from build123d import *

# Parameters (mm, degrees)
SKETCH_1_R      = 1.05
SKETCH_1_R_2    = 1.585
SKETCH_1_W      = 25
SKETCH_1_H      = 2
EXTRUDE_1_DEPTH = 2


with BuildPart() as part:
    # 草图1 → 凸台-拉伸1 (new body)
    with BuildSketch(Plane(origin=(0, 0, 0), x_dir=(1, 0, 0), z_dir=(0, 1, 0))):
        Polygon((86.47, 0), (0, 0), (0, -8.9), (-8.17, -8.9), (-8.17, -15.78), (0, -15.78), (0, -34.06), (-8.17, -34.06), (-8.17, -42.03), (0, -42.03), (0, -115), (86.47, -115), align=None)
        with Locations(Location((3, -113, 0), (0, 0, 270))):
            Circle(SKETCH_1_R, mode=Mode.SUBTRACT)
        with Locations(Location((9.47, -87.2, 0), (0, 0, 270))):
            Circle(SKETCH_1_R_2, mode=Mode.SUBTRACT)
        with Locations(Location((53.97, -87.2, 0), (0, 0, 270))):
            Circle(SKETCH_1_R_2, mode=Mode.SUBTRACT)
        with Locations(Location((66, -113, 0), (0, 0, 270))):
            Circle(SKETCH_1_R, mode=Mode.SUBTRACT)
        with Locations(Location((77.97, -101.2, 0), (0, 0, 270))):
            Circle(SKETCH_1_R_2, mode=Mode.SUBTRACT)
        with BuildLine():
            ThreePointArc((44.67, -61), (47.47, -58.2), (50.27, -61))
            Line((50.27, -61), (50.27, -69))
            ThreePointArc((50.27, -69), (47.47, -71.8), (44.67, -69))
            Line((44.67, -69), (44.67, -61))
        make_face(mode=Mode.SUBTRACT)
        with Locations(Location((9.47, -27.46, 0), (0, 0, 270))):
            Circle(SKETCH_1_R_2, mode=Mode.SUBTRACT)
        with Locations(Location((3, -2, 0), (0, 0, 270))):
            Circle(SKETCH_1_R, mode=Mode.SUBTRACT)
        with Locations((24.5, -6)):
            Rectangle(SKETCH_1_W, SKETCH_1_H, mode=Mode.SUBTRACT)
        with Locations(Location((53.97, -27.46, 0), (0, 0, 270))):
            Circle(SKETCH_1_R_2, mode=Mode.SUBTRACT)
        with Locations(Location((66, -2, 0), (0, 0, 270))):
            Circle(SKETCH_1_R, mode=Mode.SUBTRACT)
        with Locations(Location((77.97, -13.2, 0), (0, 0, 270))):
            Circle(SKETCH_1_R_2, mode=Mode.SUBTRACT)
        with Locations(Location((-4.57, -12.2, 0), (0, 0, 270))):
            Circle(SKETCH_1_R_2, mode=Mode.SUBTRACT)
        with Locations(Location((-4.07, -38.06, 0), (0, 0, 270))):
            Circle(SKETCH_1_R_2, mode=Mode.SUBTRACT)
    extrude(amount=EXTRUDE_1_DEPTH)


solid = part.part
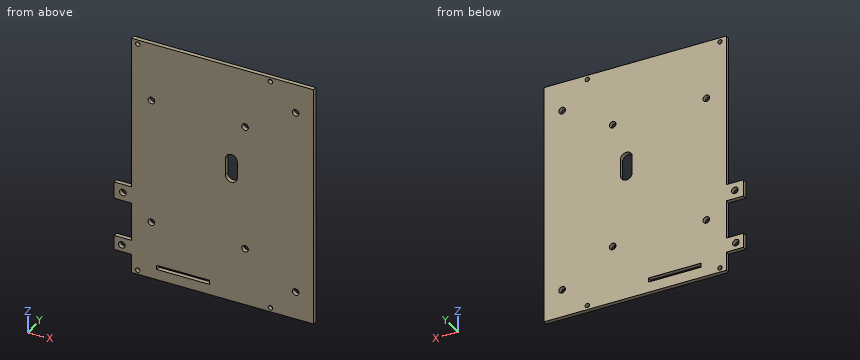
Can you work these out from the model? Positions are in its coordinate system, mm. Give positions to 0.01 mm unless a question says otherwise; leave off trailing zeros. Loops run counter-clockwise (first coordinate to the right, second up) from the corner with the lowest first, then second, coordinate; pieces in that order, holes last. Notation, with made-up numbers: (-27.5, -17.75) - (-21.5, -17.75) arc R19 cw to (-21.5, 18.25) - close; hole circle Ø9 at (46.5, 57.5). An arc over 180 degrees is marked (long way). Return JSON: item names as keys, results as strings.
1. I want a section at A-A on x = 47.47. Please give me the cut outline in (y, z), and give its area (3 significant figures).
Output values:
{"outline": "(0, 0) - (2, 0) - (2, 58.2) - (0, 58.2) - close; (0, 71.8) - (2, 71.8) - (2, 115) - (0, 115) - close", "area": "203 mm²"}
2. If I drill on line 1 (X direction, y = 0.5, z = 2); line 2 (Z direction, x = 66, y = 1.3); line 3 (X direction, y = 1.6, z = 87.2) (3 decimals), over which ranges is the centre line in solid material (lowest first)?
Output values:
{"line 1": "x = 0 to 1.95, 4.05 to 64.95, 67.05 to 86.47", "line 2": "z = 0 to 0.95, 3.05 to 111.95, 114.05 to 115", "line 3": "x = 0 to 7.885, 11.055 to 52.385, 55.555 to 86.47"}
3. I want a section at C-C on y = 0.55. Give the number of separate pieces and of enclosed holes in the cut face, and give its area (3 significant figures).
Output values:
{"separate pieces": "1", "enclosed holes": "14", "area": "9,870 mm²"}
4. I want a section at D-D on z = 31.5. Please give me the cut outline in (x, y).
Output values:
{"outline": "(0, 0) - (86.47, 0) - (86.47, 2) - (0, 2) - close"}
5. I'm going to push flat-ended pins straight in: pin 1 Ø0.6 at (y, z) = (1.5, 21.5) entering from -X; pin 2 Ø0.6 at (x, y) = (-6, 1) entering from -Z; pin 3 Ø3 at (x, z) = (77.97, 101.2) entering from -Y. Where does each tip first touch, or does it pass through?
Output values:
{"pin 1": "stops at x = 0", "pin 2": "stops at z = 8.9", "pin 3": "passes through"}
6. I want a section at B-B on z = 101.2. Please give me the cut outline in (x, y) (3 decimals), and give its area (3 significant figures).
Output values:
{"outline": "(0, 0) - (76.385, 0) - (76.385, 2) - (0, 2) - close; (79.555, 0) - (86.47, 0) - (86.47, 2) - (79.555, 2) - close", "area": "167 mm²"}
